Verification items for this drawing (mm, ordinates from the low corner). A direction names the side the tool comes from. Coordinates: 2 decimals unless noted, no trailing zeros. Loops run counter-clockwise (first coordinate to the right, second up) from the corner with the lowest first, then second, coordinate; pieces in that order, holes last. Notation, with made-up numbers: (65, 86.25) - (88, 86.25) arc R17 ccw to (88, 110.25) - close; hole circle Ø10 at (35.25, 52). An arc over 180 degrees is marked (long way). Write each question's results on one line, items separated by ' | '. Start each with the question number.
(1) Go/stop test with flat-tipped pins: pin 1 Ø12 at (y, z) = (6, 43.5) entering from +X; pin 2 Ø1.5 at (y, z) = (10.5, 34.5) entering from +X (1 decimal); pin 3 Ø8 at (x, y) = (24.5, 21) entering from -Z; pin 4 Ø5 at (y, z) = (22.5, 47) entering from -X. Record where each tip stops, or that it passes through.
(2) Sectioned sample at B-B (z = 19). Enter the section's corners in (x, y).
(3) Mould release check, pull along Z, two halves, no side actions. Record for the marked faces 1, 2 and 3: pulls with the +Z half, pulls with the -Z half, needs draft (parallel to the pull), parting line crosses it, or undercut.
(4) Sectioned sample at C-C (y = 4.5). Enter the section's corners in (x, z).
(5) Sectioned sample at A-A (x = 15). Enter the section's corners in (y, z) (1 decimal).
(6) Material ranges on probe 1 along Z at (x, y) = (15, 6); probe 2 along Z at (x, y) = (15, 16.25); probe 3 along Z at (x, y) = (25.25, 24.75), recorded low to high.
(7) Access from +Z, -Z, +X, -X, +Y, -Y to the whole of each face (thin tool, end or side, straight path). Record for the marked faces 4 and 5.
(8) Sectioned sample at D-D (x = 26.5). Enter the section's corners in (y, z).
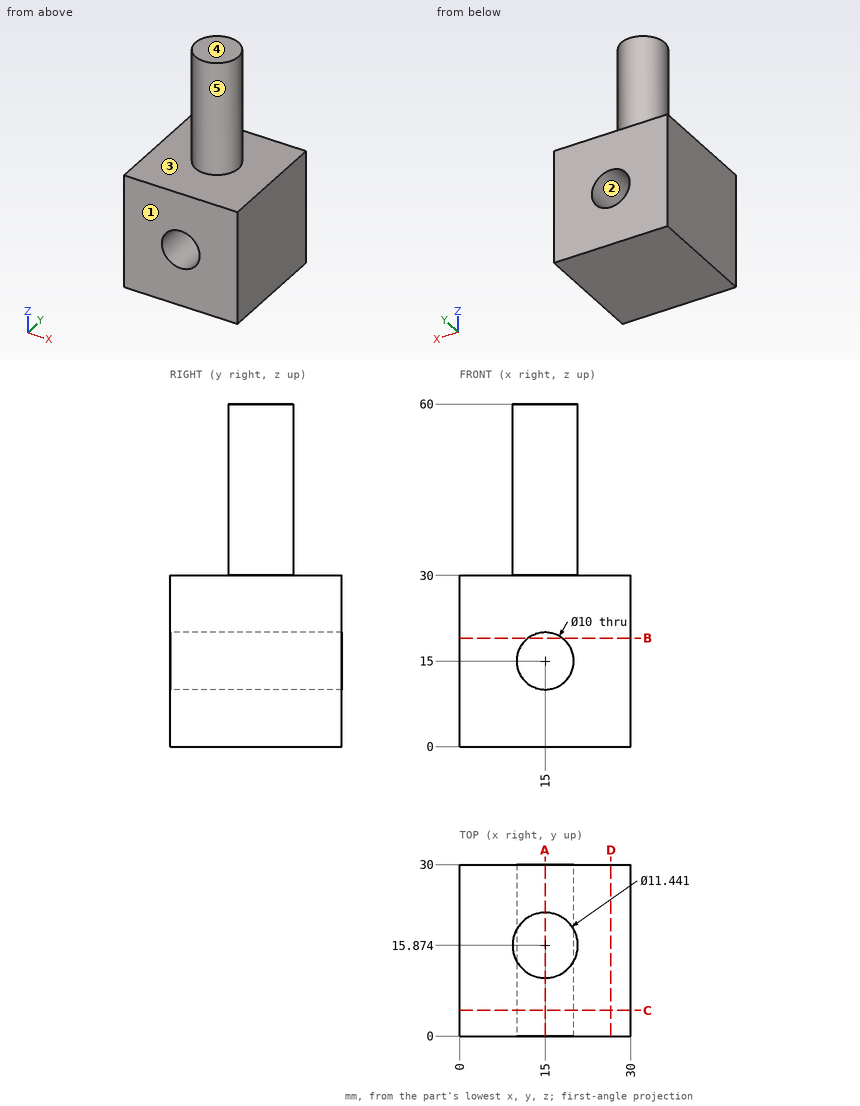
Outcome:
1) pin 1: stops at x = 19.21 | pin 2: stops at x = 18.4 | pin 3: stops at z = 0 | pin 4: stops at x = 11.04
2) outline: (0, 0) - (12, 0) - (12, 30) - (0, 30) - close; (18, 0) - (30, 0) - (30, 30) - (18, 30) - close
3) face 1: needs draft | face 2: undercut | face 3: pulls with the +Z half
4) outline: (0, 0) - (30, 0) - (30, 30) - (0, 30) - close; hole circle Ø10 at (15, 15)
5) outline: (0, 0) - (30, 0) - (30, 10) - (0, 10) - close; (0, 20) - (30, 20) - (30, 30) - (21.6, 30) - (21.6, 60) - (10.2, 60) - (10.2, 30) - (0, 30) - close
6) probe 1: z = 0 to 10, 20 to 30 | probe 2: z = 0 to 10, 20 to 60 | probe 3: z = 0 to 30
7) face 4: +Z, +X, -X, +Y, -Y | face 5: +Z
8) outline: (0, 0) - (30, 0) - (30, 30) - (0, 30) - close
